Can you work these out from the drawing? Everything is in mm from the part's minimum corner. A direction names the side the tool comes from. Give positions to 0.01 mm unless a question says otherwise; leave off trailing zeros. Order: outer loops, then holes, each group sorted by start corner. A loop starts at its lowest first (then second) coordinate and runs counter-clockwise, first axis right, second up. Notation, with made-up numbers: (61.25, 27) - (112.25, 27) arc R9 ccw to (112.25, 44) - close; hole circle Ø3 at (73, -29.5). An arc over 180 degrees is marked (long way). One line per question, with ' | ' between items.
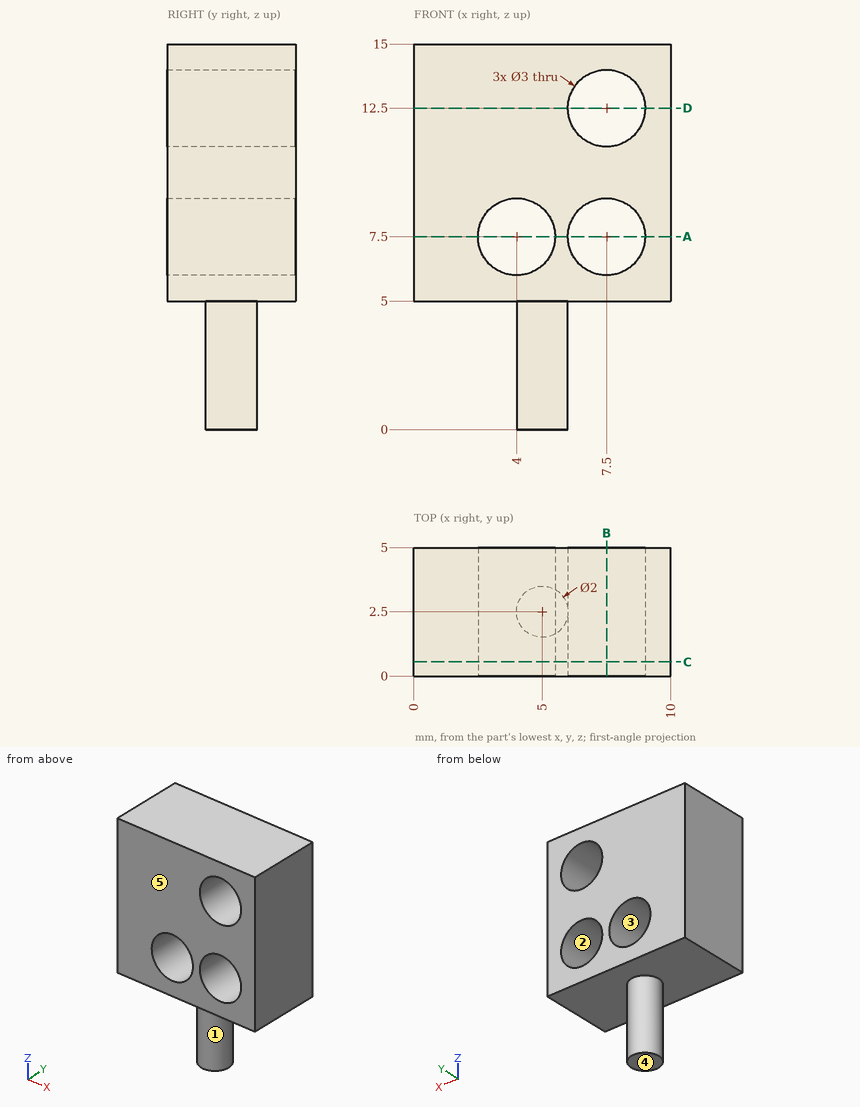
(1) Imagine slicing it at A-A (z = 7.5). List the corners of the cut face in (x, y) for me.
Answer below:
outline: (0, 0) - (2.5, 0) - (2.5, 5) - (0, 5) - close; (5.5, 0) - (6, 0) - (6, 5) - (5.5, 5) - close; (9, 0) - (10, 0) - (10, 5) - (9, 5) - close
(2) Will this pin go through, and if not, where does the flat tip stop? pin 1 (1 mm diameter, centred on x = 4, y = 4, fed in from -Z).
Answer below:
pin 1: z = 5
(3) Imagine slicing it at B-B (x = 7.5). List the corners of the cut face in (y, z) for me.
Answer below:
outline: (0, 5) - (5, 5) - (5, 6) - (0, 6) - close; (0, 9) - (5, 9) - (5, 11) - (0, 11) - close; (0, 14) - (5, 14) - (5, 15) - (0, 15) - close
(4) Imagine slicing it at D-D (z = 12.5). List the corners of the cut face in (x, y) for me.
Answer below:
outline: (0, 0) - (6, 0) - (6, 5) - (0, 5) - close; (9, 0) - (10, 0) - (10, 5) - (9, 5) - close
(5) If we mould it in two halves opening along Z, with no side actions, what happens to the marked faces 3, 4 and 5? For each: released by +Z, released by -Z, zero draft, split by the parting line, or undercut.
Answer below:
face 3: undercut | face 4: released by -Z | face 5: zero draft
(6) Imagine slicing it at C-C (y = 0.55). List the corners of the cut face in (x, z) for me, and give its area (3 significant figures).
Answer below:
outline: (0, 5) - (10, 5) - (10, 15) - (0, 15) - close; hole circle Ø3 at (4, 7.5); hole circle Ø3 at (7.5, 7.5); hole circle Ø3 at (7.5, 12.5) | area: 78.8 mm^2
(7) On a 3-axis mill with a long thin cutter (end or side, diameter ignored), from which of +Z, -Z, +X, -X, +Y, -Y can I reach the whole of each face in a straight line? I mean the marked faces 1 and 2. Say none if no direction works.
Answer below:
face 1: -Z | face 2: +Y, -Y
(8) If I drill on line 1 (X direction, y = 1.55, z = 7.5); line 2 (X direction, y = 2.9, z = 12.5); line 3 (Z direction, x = 8.5, y = 3.75), over which ranges is the centre line in solid material (lowest first)?
Answer below:
line 1: 0 to 2.5, 5.5 to 6, 9 to 10 | line 2: 0 to 6, 9 to 10 | line 3: 5 to 6.38, 8.62 to 11.38, 13.62 to 15
